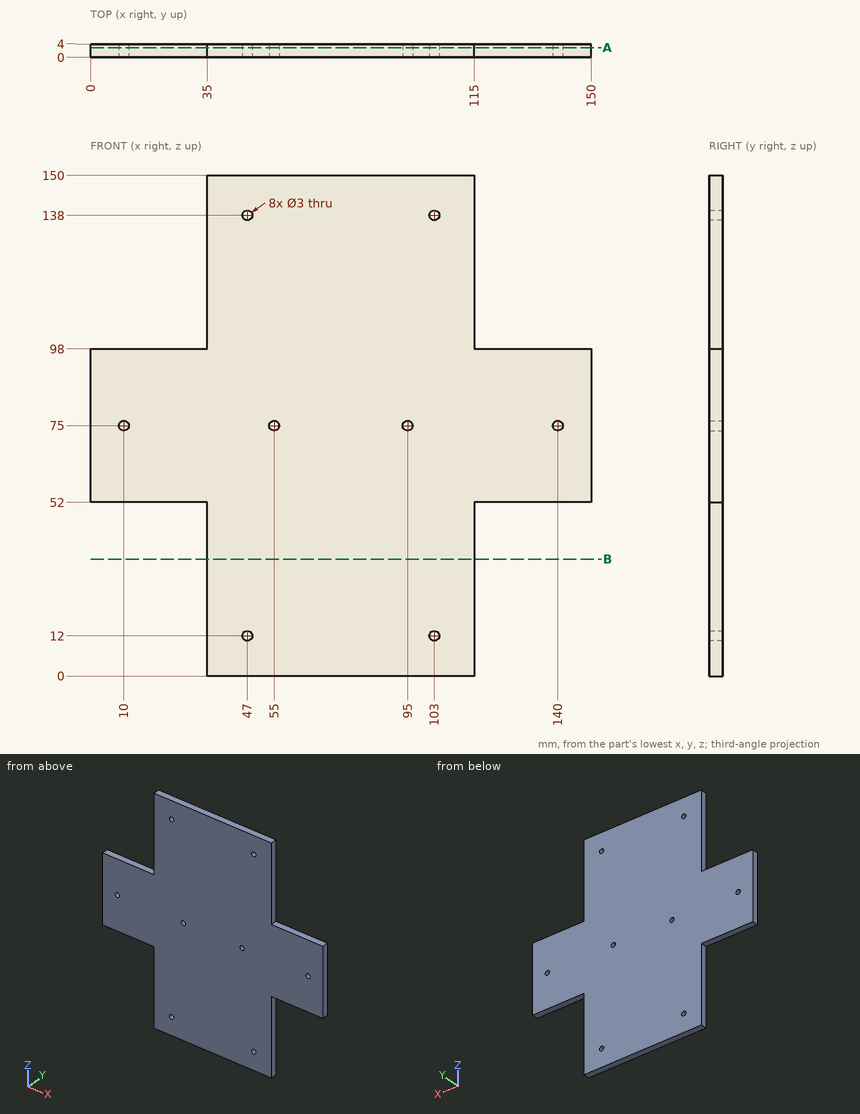
Input: dimensioned drawing with shaded views. Units: mm. Origin: part minimum x, y, z. Coordinates: 2 decimals unless noted, no trailing zeros. Write each loop counter-clockwise with the first axis right and the second up, starting at its lowest first coordinate (ties: lowest second). Pieces come first, ordered by that corner, then holes. Notation, with made-up numbers: M 78.5,54 L 87.5,54 A25 cw 87.5,75 Z; hole C 61.5,-8.5 d10. An arc over 180 degrees is marked long. Use a Markdown table: item, result.
1) First-contact query: pin 1 Ø2.5 at (x, z) = (47, 12) entering from +Y; pin 2 Ø2 at (y, z) = (1, 16.5) entering from +X; pin 3 Ø2 at (x, y) = (20.5, 2.5) entering from +Z. Flat tips, straight axial feed; report the tip coordinate or a pass-through.
Conclusion:
| item | result |
|---|---|
| pin 1 | passes through |
| pin 2 | stops at x = 115 |
| pin 3 | stops at z = 98 |
2) Section A-A, the plane y = 2.9. Give the number of separate pieces and of enclosed holes in the cut face, then the cut area to 3 significant figures.
Conclusion:
| item | result |
|---|---|
| separate pieces | 1 |
| enclosed holes | 8 |
| area | 15,200 mm^2 |
3) Section B-B, the plane z = 35. Output: boundary loops of the cut face in (x, y), then the cut area to 3 significant figures.
Conclusion:
| item | result |
|---|---|
| outline | M 35,0 L 115,0 L 115,4 L 35,4 Z |
| area | 320 mm^2 |
4) Ray query, L1, parallel to X at y = 3.2, z = 75; L2, parallel to Z at x = 95, y = 2.25; L3, parallel to Z at x = 47, y = 2.45. Return the intervals inside material, ascending.
Conclusion:
| item | result |
|---|---|
| L1 | x = 0 to 8.5, 11.5 to 53.5, 56.5 to 93.5, 96.5 to 138.5, 141.5 to 150 |
| L2 | z = 0 to 73.5, 76.5 to 150 |
| L3 | z = 0 to 10.5, 13.5 to 136.5, 139.5 to 150 |
